Geometry: final body of the model. Coordinates: model frame, mm. Face numbers are marked on the shaded views. Give positions to 0.01 mm unless a question says otherwise; leave off trailing zeros. Loops run counter-clockwise (first coordinate to the right, second up) from the corner with the lowest first, then second, coordinate; pieces in that order, holes last. Notation, with made-up numbers: M 74.5,68.5 L 129.5,68.5 A23 ccw 129.5,90.5 Z; hole C -15,79 d9. An arc over 180 degrees is marked long. Put each result on its own line as item: value.
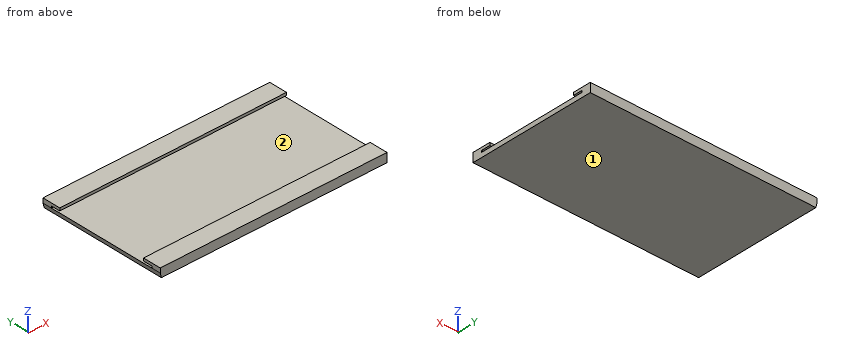
```python
from build123d import *

# Parameters (mm, degrees)
BOSS_EXTRUDE1_DEPTH      = 5
BOSS_EXTRUDE1_DEPTH_BACK = 5
SKETCH1_W                = 250
SKETCH1_H                = 10
SKETCH1_H_2              = 100
SKETCH1_3_W              = 250
SKETCH1_3_H              = 100
CUT_EXTRUDE1_DEPTH       = 260.663243452
SKETCH1_4_W              = 250
SKETCH1_4_H              = 10
CUT_EXTRUDE2_DEPTH       = 2
CUT_EXTRUDE3_DEPTH       = 260.663243452
CUT_EXTRUDE3_DEPTH_BACK  = 260.663243452


with BuildPart() as part:
    # Sketch1 → Boss-Extrude1 (new, two sides: drawn at the far end of the back side and taken through both)
    with BuildSketch(Plane.XY.offset(-BOSS_EXTRUDE1_DEPTH_BACK)):
        with Locations((125, 55)):
            Rectangle(SKETCH1_W, SKETCH1_H)
        with Locations((125, 65)):
            Rectangle(SKETCH1_W, SKETCH1_H)
        with Locations((125, -55)):
            Rectangle(SKETCH1_W, SKETCH1_H)
        with Locations((125, -65)):
            Rectangle(SKETCH1_W, SKETCH1_H)
        with Locations((125, 0)):
            Rectangle(SKETCH1_W, SKETCH1_H_2)
    extrude(amount=BOSS_EXTRUDE1_DEPTH + BOSS_EXTRUDE1_DEPTH_BACK)

    # Sketch1_3 → Cut-Extrude1 (cut, through all)
    with BuildSketch(Plane.XY):
        with Locations((125, 0)):
            Rectangle(SKETCH1_3_W, SKETCH1_3_H)
    extrude(amount=CUT_EXTRUDE1_DEPTH, mode=Mode.SUBTRACT)

    # Sketch1_4 → Cut-Extrude2 (cut)
    with BuildSketch(Plane.XY):
        with Locations((125, 55)):
            Rectangle(SKETCH1_4_W, SKETCH1_4_H)
        with Locations((125, -55)):
            Rectangle(SKETCH1_4_W, SKETCH1_4_H)
    extrude(amount=CUT_EXTRUDE2_DEPTH, mode=Mode.SUBTRACT)

    # Sketch2 → Cut-Extrude3 (cut, two sides: drawn at the far end of the back side and taken through both)
    with BuildSketch(Plane(origin=(0, 0, 0), x_dir=(1, 0, 0), z_dir=(0, 1, 0)).offset(-CUT_EXTRUDE3_DEPTH_BACK)):
        Polygon((0, 0), (7.5, 30), (0, 30), align=None)
    extrude(amount=CUT_EXTRUDE3_DEPTH + CUT_EXTRUDE3_DEPTH_BACK, mode=Mode.SUBTRACT)


solid = part.part
```
Item 1: Mould query, pull axis Y, two halves, no side actions, for the marked faces 1 and 2. Classes: pulls with the +Y half, pulls with the -Y half, needs draft (parallel to the pull), parting line crosses it, or undercut.
Output values:
face 1: needs draft
face 2: undercut
Item 2: Section B-B on x = 218.5. Output: boundary loops of the cut face in (y, z).
Output values:
outline: M -70,-5 L 70,-5 L 70,5 L 50,5 L 50,2 L 60,2 L 60,0 L -60,0 L -60,2 L -50,2 L -50,5 L -70,5 Z
Item 3: Section A-A on y = -56.5. Output: boundary loops of the cut face in (x, z).
Output values:
outline: M 0,0 L 1.25,-5 L 250,-5 L 250,0 Z; M 0,2 L 250,2 L 250,5 L 0,5 Z
Item 4: Line query: probe 1 along Y at (x, z) = (26, 3.5); probe 2 along Y at (x, z) = (75.5, 1.25); probe 3 along Z at (x, y) = (159, 54). Output: solid intervals per line, ascending. Write a range as [from, to].
Output values:
probe 1: [-70, -50], [50, 70]
probe 2: [-70, -60], [60, 70]
probe 3: [-5, 0], [2, 5]
